```python
from build123d import *

# Parameters (mm, degrees)
BOSS_EXTRUDE1_DEPTH = 31
BOSS_EXTRUDE2_START = 22
BOSS_EXTRUDE2_DEPTH = 9
BOSS_EXTRUDE4_START = -22
BOSS_EXTRUDE4_DEPTH = 9


with BuildPart() as part:
    # Sketch1 → Boss-Extrude1 (new, symmetric)
    with BuildSketch(Plane(origin=(0, 0, 0), x_dir=(0, 0, -1), z_dir=(1, 0, 0))):
        Polygon((-33.203112203, -21.939393939), (-33.203112203, 20.060606061), (-13.203112203, 20.060606061), (-13.203112203, -5.939393939), (16.796887797, -5.939393939), (16.796887797, -21.939393939), (0.796887797, -21.939393939), (0.796887797, -15.939393939), (-17.203112203, -15.939393939), (-17.203112203, -21.939393939), align=None)
    extrude(amount=BOSS_EXTRUDE1_DEPTH, both=True)

    # Sketch1_4 → Boss-Extrude2 (add)
    with BuildSketch(Plane(origin=(0, 0, 0), x_dir=(0, 0, -1), z_dir=(1, 0, 0)).offset(BOSS_EXTRUDE2_START)):
        Polygon((-13.203112203, 20.060606061), (16.796887797, -5.939393939), (-13.203112203, -5.939393939), align=None)
    extrude(amount=BOSS_EXTRUDE2_DEPTH)

    # Sketch1_14 → Boss-Extrude4 (add)
    with BuildSketch(Plane(origin=(0, 0, 0), x_dir=(0, 0, -1), z_dir=(1, 0, 0)).offset(BOSS_EXTRUDE4_START)):
        Polygon((-13.203112203, 20.060606061), (16.796887797, -5.939393939), (-13.203112203, -5.939393939), align=None)
    extrude(amount=-BOSS_EXTRUDE4_DEPTH)


solid = part.part
```
Here's how the part is built. I have some questions about the finished solid (model axes, mm). A direction names the side the tool comes from. Give positions to 0.01 mm unless a question says otherwise; leave off trailing zeros. Loops run counter-clockwise (first coordinate to the right, second up) from the corner with the lowest first, then second, coordinate; pieces in that order, holes last. Notation, with made-up numbers: (82.5, 68) -> (116.5, 68) arc R34 cw to (116.5, 107) -> close; hole circle Ø4 at (41.25, 70.5). An arc over 180 degrees is marked (long way). Use one line per item in the form item = value. Start each with the question number.
1) Please list where these lines run through material, in increasing order: line 1 along Z through (x, y) = (15, -17.5); line 2 along Z through (x, y) = (21.5, 8.5); line 3 along Y through (x, z) = (-3.5, -10.5).
2) Imagine slicing it at C-C (y = -4). Please give me the cut outline in (x, z), then the cut area to 3 significant figures.
3) Thinking about a two-plate mould opening in X: for faces 1 (the face through (-31, -1, 13)), 2 (the face through (0, -15.939, 8)), 3 (the face through (0, 7, 13.203)), which applies, +X half, -X half, draft (parallel to the pull), parting line (faces both ways), or undercut?
4) For P1, Ø12, axis at x = 9.5, y = 8.5, coming from the -Z side; P2, Ø8, axis at x = -3.5, z = 1.5, coming from the +Y side, each with a flat end and sliding along its axis, tell me the tip position at first contact or that it passes through.
5) Imagine slicing it at A-A (x = 4). Please give me the cut outline in (y, z), then the cut area to 3 significant figures.
6) Imagine slicing it at D-D (z = 16). Please give me the cut outline in (x, y).
7) Imagine slicing it at B-B (z = -7.5). Please give me the cut outline in (x, y).
8) Which directions (+Z, -Z, +X, -X, +Y, -Y) give clear straight access to the entire face, cutting with the end or side of a thin tool? Please do faces 4 (the face through (0, -5.939, -2)), 5 (the face through (0, -21.939, -9)), 6 (the face through (0, -19, -0.797)).
Check values:
q1.line_1 = -16.8 to -0.8, 17.2 to 33.2
q1.line_2 = 13.2 to 33.2
q1.line_3 = -21.94 to -5.94
q2.outline = (-31, -14.56) -> (-22, -14.56) -> (-22, 13.2) -> (22, 13.2) -> (22, -14.56) -> (31, -14.56) -> (31, 33.2) -> (-31, 33.2) -> close
q2.area = 1,740 mm^2
q3.face_1 = -X half
q3.face_2 = draft
q3.face_3 = undercut
q4.P1 = 13.2
q4.P2 = -5.94
q5.outline = (-21.94, -16.8) -> (-5.94, -16.8) -> (-5.94, 13.2) -> (20.06, 13.2) -> (20.06, 33.2) -> (-21.94, 33.2) -> (-21.94, 17.2) -> (-15.94, 17.2) -> (-15.94, -0.8) -> (-21.94, -0.8) -> close
q5.area = 1,210 mm^2
q6.outline = (-31, -15.94) -> (31, -15.94) -> (31, 20.06) -> (-31, 20.06) -> close
q7.outline = (-31, -21.94) -> (31, -21.94) -> (31, 2.12) -> (22, 2.12) -> (22, -5.94) -> (-22, -5.94) -> (-22, 2.12) -> (-31, 2.12) -> close
q8.face_4 = -Z, +Y
q8.face_5 = +Z, -Z, +X, -X, -Y
q8.face_6 = +X, -X, -Y
